For this review, take the finished solid that the model builds, in its own axes (mm). Coordinates: 2 decimals unless noted, no trailing zeros. Order: outer loops, then holes, each group sorted by start corner. A loop starts at its lowest first (then second) coordinate and runs counter-clockwise, first axis right, second up. Notation, with made-up numbers: (59, 34.5) -> (70, 34.5) arc R24 cw to (70, 67.5) -> close; hole circle Ø5 at (29, 1). An arc over 180 degrees is marked (long way). Write item = value, one per line. Start each with the question number.
1) Consider section B-B on z = 0. Give the boundary of the cut face in (x, y).
2) Consider section C-C on y = 2.45. Give the boundary of the cut face in (x, z), and give its area (3 significant figures).
3) Consider section A-A on x = 52.5. Give the boundary of the cut face in (y, z).
4) Wall thickness on probe 1 along X at (y, z) = (2.3, -32.5); probe 2 along Z at (x, y) = (-52.5, 1.75); probe 3 along X at (y, z) = (2.7, 33.5): over which ranges is each line inside the solid? List them lowest first. Write a range as [from, to].
5) Draft analysis for pull direction Z (two halves, no side actions). For faces 1 (the face through (-1, 1, 40)), 2 (the face through (-28, 0, -1)), 3 (the face through (53.84, 1.52, -34.61)), state which applies: +Z half, -Z half, draft (parallel to the pull), parting line (faces both ways), or undercut.
6) Insertion check: pin 1 Ø3 at (x, z) = (-24.5, -1.5) entering from -Y. The pin has a flat end and moves straight along its axis. Give the tip position at first contact, or say it passes through.
7) Consider section D-D on z = -32.5. Give the boundary of the cut face in (x, y), and give its area (3 significant figures).
from build123d import *

# Parameters (mm, degrees)
SKETCH1_R                       = 26.5
SKETCH1_W                       = 15
SKETCH1_H                       = 15
BOSS_EXTRUDE1_DEPTH             = 3
TAP_DRILL_FOR_M6X1_0_TAP1_D     = 5
TAP_DRILL_FOR_M6X1_0_TAP1_DEPTH = 3


with BuildPart() as part:
    # Sketch1 → Boss-Extrude1 (new body)
    with BuildSketch(Plane(origin=(0, 0, 0), x_dir=(1, 0, 0), z_dir=(0, 1, 0))):
        Polygon((45, 40), (-45, 40), (-45, 25), (-60, 25), (-60, -25), (-45, -25), (-45, -40), (45, -40), (45, -25), (60, -25), (60, 25), (45, 25), align=None)
        Circle(SKETCH1_R, mode=Mode.SUBTRACT)
        with Locations((52.5, -32.5)):
            Rectangle(SKETCH1_W, SKETCH1_H)
        with Locations((52.5, 32.5)):
            Rectangle(SKETCH1_W, SKETCH1_H)
        with Locations((-52.5, 32.5)):
            Rectangle(SKETCH1_W, SKETCH1_H)
        with Locations((-52.5, -32.5)):
            Rectangle(SKETCH1_W, SKETCH1_H)
    extrude(amount=BOSS_EXTRUDE1_DEPTH)

    # Tap Drill for M6x1.0 Tap1
    with Locations(Plane(origin=(0, 0, 0), x_dir=(-1, 0, 0), z_dir=(0, -1, 0))):
        with Locations((52.5, -32.5), (-52.5, -32.5), (-52.5, 32.5), (52.5, 32.5)):
            Hole(TAP_DRILL_FOR_M6X1_0_TAP1_D / 2, depth=TAP_DRILL_FOR_M6X1_0_TAP1_DEPTH)


solid = part.part
Answer sheet:
q1.outline = (-60, 0) -> (-26.5, 0) -> (-26.5, 3) -> (-60, 3) -> close; (26.5, 0) -> (60, 0) -> (60, 3) -> (26.5, 3) -> close
q2.outline = (-60, -40) -> (60, -40) -> (60, 40) -> (-60, 40) -> close; hole circle Ø5 at (-52.5, -32.5); hole circle Ø5 at (-52.5, 32.5); hole circle Ø53 at (0, 0); hole circle Ø5 at (52.5, -32.5); hole circle Ø5 at (52.5, 32.5)
q2.area = 7,320 mm2
q3.outline = (0, -40) -> (3, -40) -> (3, -35) -> (0, -35) -> close; (0, -30) -> (3, -30) -> (3, 30) -> (0, 30) -> close; (0, 35) -> (3, 35) -> (3, 40) -> (0, 40) -> close
q4.probe_1 = [-60, -55], [-50, 50], [55, 60]
q4.probe_2 = [-40, -35], [-30, 30], [35, 40]
q4.probe_3 = [-60, -54.79], [-50.21, 50.21], [54.79, 60]
q5.face_1 = +Z half
q5.face_2 = draft
q5.face_3 = undercut
q6.pin_1 = through
q7.outline = (-60, 0) -> (-55, 0) -> (-55, 3) -> (-60, 3) -> close; (-50, 0) -> (50, 0) -> (50, 3) -> (-50, 3) -> close; (55, 0) -> (60, 0) -> (60, 3) -> (55, 3) -> close
q7.area = 330 mm2
